from build123d import *

# Parameters (mm, degrees)
MODEL_R             = 5.191903136
MODEL_R_2           = 5.25
BOSS_EXTRUDE1_DEPTH = 5
SKETCH3_R           = 45.25
CUT_EXTRUDE1_DEPTH  = 6


with BuildPart() as part:
    # Model → Boss-Extrude1 (new body)
    with BuildSketch(Plane.XY):
        with BuildLine():
            Line((869.6, 129.800004709), (854.6, 129.800004709))
            Line((854.6, 129.800004709), (854.6, 124.800004709))
            ThreePointArc((854.6, 124.800004709), (842.940279, 95.005240735), (815.123335737, 79.19718198))
            ThreePointArc((815.123335737, 79.19718198), (819.577050566, 70.004649675), (820.028101645, 59.800004709))
            Line((820.028101645, 59.800004709), (849.60000149, 59.800004709))
            ThreePointArc((849.60000149, 59.800004709), (852.428428615, 58.628431833), (853.60000149, 55.800004709))
            Line((853.60000149, 55.800004709), (853.60000149, 44.400154403))
            Line((853.60000149, 44.400154403), (856.099999799, 43.300004388))
            Line((856.099999799, 43.300004388), (853.60000149, 38.829377357))
            Line((853.60000149, 38.829377357), (853.60000149, -2.199993903))
            Line((853.60000149, -2.199993903), (869.6, -2.199993903))
            Line((869.6, -2.199993903), (869.6, 129.800004709))
        make_face()
        with Locations((861.6, 9.391497171)):
            Circle(MODEL_R, mode=Mode.SUBTRACT)
        with Locations((861.6, 114.800004709)):
            Circle(MODEL_R_2, mode=Mode.SUBTRACT)
    extrude(amount=BOSS_EXTRUDE1_DEPTH)

    # Sketch3 → Cut-Extrude1 (cut)
    with BuildSketch(Plane(origin=(0, 0, 0), x_dir=(-1, 0, 0), z_dir=(0, 0, -1))):
        with Locations((-795.076378777, 63.809415284)):
            Circle(SKETCH3_R)
    extrude(amount=-CUT_EXTRUDE1_DEPTH, mode=Mode.SUBTRACT)


solid = part.part
Can you work these out from the model? Positions are in its coordinate system, mm. A direction names the side the tool comes from. Coordinates: 2 decimals unless noted, no trailing zeros. Loops run counter-clockwise (first coordinate to the right, second up) from the corner with the lowest first, then second, coordinate; pieces in that order, holes last. Notation, with made-up numbers: M 13,39.25 L 19,39.25 A7 ccw 19,45.25 Z; hole C 54.5,3.5 d6. An arc over 180 degrees is marked long. Answer as CSV lines item,"result". Start each with the question number.
1. Suppose I cut it at A-A, the plane x = 861.6. List the corners of the cut face in (y, z) for me.
2. Suppose I cut it at D-D, the plane x = 838. List the corners of the cut face in (y, z) for me, plus the area to 3 significant figures.
3. Suppose I cut it at B-B, the plane z = 3.6. List the corners of the cut face in (x, y) for me.
4. Suppose I cut it at C-C, the plane y = 46.5. List the corners of the cut face in (x, z) for me, plus the area to 3 significant figures.
5. For faces 1 (the face through (854.87, 41.1, 2.46)), 2 (the face through (859, 65, 5)), 3 (the face through (854.6, 127, 2)), 4 (the face through (853.6, 19, 2)), which set-ups out of +Z, -Z, +X, -X, +Y, -Y let a thin tool reach every point of the face, with its end or its side?
6. For pin 1 Ø2.5 at (y, z) = (17, 2.5) entering from -X; pin 2 Ø1.5 at (y, z) = (115.5, 4.5) entering from -X; pin 3 Ø1.5 at (y, z) = (127.5, 2.5) entering from -X, each with a flat end and sliding along its axis, tell me the tip position at first contact or that it passes through.
7. Thinking about a two-plate mould opening in Y: for faces 5 (the face through (857.43, 111.61, 2.46)), 6 (the face through (859, 65, 0)), 7 (the face through (845, 59.8, 2)), which applies, +Y half, -Y half, draft (parallel to the pull), parting line (faces both ways), or undercut?
8. If I drill on probe 1 along Y at (x, z) = (861.6, 1.15); probe 2 along Y at (x, z) = (864.5, 3.1) (3 decimals); probe 3 along Y at (x, z) = (855, 0.25), over which ranges is the centre line in solid material (lowest first)? Write a range as [from, to].
Output:
1,outline,"M -2.2,0 L 4.2,0 L 4.2,5 L -2.2,5 Z; M 14.58,0 L 109.55,0 L 109.55,5 L 14.58,5 Z; M 120.05,0 L 129.8,0 L 129.8,5 L 120.05,5 Z"
2,outline,"M 78.13,0 L 90.08,0 L 90.08,5 L 78.13,5 Z"
2,area,"59.7 mm^2"
3,outline,"M 833.96,86.95 A45.25 cw 840.15,59.8 L 849.6,59.8 A4 cw 853.6,55.8 L 853.6,44.4 L 856.1,43.3 L 853.6,38.83 L 853.6,-2.2 L 869.6,-2.2 L 869.6,129.8 L 854.6,129.8 L 854.6,124.8 A47.9 cw Z; hole C 861.6,114.8 d10.5; hole C 861.6,9.39 d10.38"
4,outline,"M 853.6,0 L 869.6,0 L 869.6,5 L 853.6,5 Z"
4,area,"80.0 mm^2"
5,face 1,"+Z, -Z, -X"
5,face 2,"+Z, +X, -X, +Y, -Y"
5,face 3,"+Z, -Z, -X, +Y"
5,face 4,"+Z, -Z, -X, -Y"
6,pin 1,"stops at x = 853.6"
6,pin 2,"stops at x = 853.2"
6,pin 3,"stops at x = 854.6"
7,face 5,"undercut"
7,face 6,"draft"
7,face 7,"-Y half"
8,probe 1,"y = [-2.2, 4.2], [14.58, 109.55], [120.05, 129.8]"
8,probe 2,"y = [-2.2, 5.085], [13.698, 110.424], [119.176, 129.8]"
8,probe 3,"y = [-2.2, 41.33], [43.78, 129.8]"
